from build123d import *

# Parameters (mm, degrees)
SKETCH_1_R      = 1
EXTRUDE_1_DEPTH = 1


with BuildPart() as part:
    # 草图1 → 凸台-拉伸1 (new body)
    with BuildSketch(Plane(origin=(0, 0, 0), x_dir=(1, 0, 0), z_dir=(0, 1, 0))):
        with BuildLine():
            Line((-5.75, -9.959292144), (-4.58121163, -7.934891304))
            ThreePointArc((-4.58121163, -7.934891304), (-4.960583519, -5.355685993), (-7.558022947, -5.1331293))
            ThreePointArc((-7.558022947, -5.1331293), (-8.587203168, -5.274503777), (-9.341056075, -4.559727963))
            ThreePointArc((-9.341056075, -4.559727963), (0, 9), (9.341056075, -4.559727963))
            ThreePointArc((9.341056075, -4.559727963), (8.587203168, -5.274503777), (7.558022947, -5.1331293))
            ThreePointArc((7.558022947, -5.1331293), (4.960583519, -5.355685993), (4.58121163, -7.934891304))
            Line((4.58121163, -7.934891304), (5.75, -9.959292144))
            ThreePointArc((5.75, -9.959292144), (0, 11.5), (-5.75, -9.959292144))
        make_face()
        with Locations(Location((-6.399864978, -6.884891304, 0), (0, 0, 270))):
            Circle(SKETCH_1_R, mode=Mode.SUBTRACT)
        with Locations(Location((6.399864978, -6.884891304, 0), (0, 0, 270))):
            Circle(SKETCH_1_R, mode=Mode.SUBTRACT)
    extrude(amount=EXTRUDE_1_DEPTH)


solid = part.part
Geometry check sheet. Reference: the model listing, model coordinates, mm. A direction names the side the tool comes from. Give positions to 0.01 mm unless a question says otherwise; leave off trailing zeros. Loops run counter-clockwise (first coordinate to the right, second up) from the corner with the lowest first, then second, coordinate; pieces in that order, holes last.
(1) Release check for a two-part mould opening along Z. For faces 4 (the flat face through (5.157, 0.493, 8.933)), 5 (the cylindrical face through (-4.932, 0.493, 5.383)), 6 (the flat face through (0, 1, -10)) record: released by +Z, released by -Z, zero draft, split by the parting line, or undercut.
From the geometry:
face 4: released by +Z
face 5: undercut
face 6: zero draft
(2) Set-up check for faces 1 (the flat face through (-5.174, 0.493, 8.961)), 2 (the flat face through (0, 0, -10)), 3 (the cylindrical face through (-8.57, 0.49, 5.28)): record each of +Z, -Z, +X, -X, +Y, -Y from which the full face is reachable in a straight line by a thin tool's end or side.
From the geometry:
face 1: +Z, +Y, -Y
face 2: +Z, -Z, +X, -X, -Y
face 3: +Y, -Y
(3) Thickness scan on L1, parallel to Z at x = -6, y = 0.1; L2, parallel to Z at x = 7.25, y = 0.6; L3, parallel to X at y = 0.25, z = 6.75. Record the ranges inside material, lowest first.
From the geometry:
L1: z = -9.81 to -7, 4.82 to 5.97, 7.8 to 9.81
L2: z = -8.93 to -5.89, 4.96 to 6.36, 7.41 to 8.93
L3: x = -9.31 to -7.39, -5.41 to -4.3, 4.3 to 5.41, 7.39 to 9.31
(4) Section check B-B on z = 0. Record the cut outline in (x, y), then the cut area to 3 significant figures.
From the geometry:
outline: (-11.5, 0) - (-9.95, 0) - (-9.95, 1) - (-11.5, 1) - close; (9.95, 0) - (11.5, 0) - (11.5, 1) - (9.95, 1) - close
area: 3.11 mm2
(5) Section check D-D on x = 0. Record the cut outline in (y, z).
From the geometry:
outline: (0, -11.5) - (1, -11.5) - (1, -9) - (0, -9) - close
(6) Section check A-A on x = 5. Record the cut outline in (y, z).
From the geometry:
outline: (0, -10.36) - (1, -10.36) - (1, -7.66) - (0, -7.66) - close; (0, 5.32) - (1, 5.32) - (1, 8.66) - (0, 8.66) - close
(7) Section check C-C on y = 0.5. Record the cut outline in (x, z), then the cut area to 3 significant figures.
From the geometry:
outline: (-9.34, 4.56) arc R1.2 cw to (-7.56, 5.13) arc R2.1 ccw to (-4.58, 7.93) - (-5.75, 9.96) arc R11.5 ccw (long way) to (5.75, 9.96) - (4.58, 7.93) arc R2.1 ccw to (7.56, 5.13) arc R1.2 cw to (9.34, 4.56) arc R10 cw (long way) to start; hole circle Ø2 at (-6.4, 6.88); hole circle Ø2 at (6.4, 6.88)
area: 115 mm2
